Geometry check sheet. Reference: the model listing, model coordinates, mm. Round coordinates to 2 decimals unless told otherwise and drop trailing zeros. Write each loop counter-clockwise with the first axis right and the second up, starting at its lowest first coordinate (ties: lowest second). Pieces come first, ordered by that corner, then holes. Notation, with made-up numbers: M 40,-7 L 68,-7 A18 cw 68,18 Z; hole C 77,11.25 d4. An arc over 180 degrees is marked long. Put each result on its own line as item: value. Start each with the question number.
(1) Section check A-A on x = -110. Record the cut outline in (y, z).
(2) Gauge pin test, flat ends, axial feed: pin 1 (2.5 mm diameter, centred on x = 186, y = -15, fed in from -Z); pin 2 (0.8 mm diameter, centred on y = -16.5, z = 3, fed in from +X); pin 3 (1.2 mm diameter, centred on y = -9.5, z = -4.5, fed in from -X). Record the tip position at first contact, or that the pin passes through.
(3) Material ranges on probe 1 along X at (y, z) = (-21, 2); probe 2 along Y at (x, z) = (120, -0.75), recorded low to high.
from build123d import *

# Parameters (mm, degrees)
F1_DEPTH      = 35
F2_W          = 3
F2_H          = 3
F3_DEPTH      = 187.5
F3_DEPTH_BACK = 187.5


with BuildPart() as f1:
    # F0 (on Front) → F1 (new body)
    with BuildSketch(Plane.XZ):
        Polygon((-226.934456, 2.5), (-226.934456, 0), (-226.934456, -2.5), (-221.934456, -2.5), (-221.934456, -5), (153.065544, -5), (153.065544, -2.5), (158.065544, -2.5), (158.065544, 2.5), (153.065544, 2.5), (153.065544, 5), (-221.934456, 5), (-221.934456, 2.5), align=None)
    extrude(amount=F1_DEPTH)


with BuildPart() as f3:
    # F2 (on Right) → F3 (new body, two sides)
    with BuildSketch(Plane.YZ) as f3_sk:
        with Locations((-32.222062, -1.036781)):
            Rectangle(F2_W, F2_H)
    extrude(amount=F3_DEPTH)
    extrude(f3_sk.sketch, amount=-F3_DEPTH_BACK)


with BuildPart() as f1_1:
    # F4: moved
    add(f1.part.moved(Location((29.4, 1.4, -1))))

    # F5: cut F3
    add(f3.part, mode=Mode.SUBTRACT)


solid = f1_1.part
Answers follow:
1. outline: M -33.6,-6 L 1.4,-6 L 1.4,4 L -33.6,4 L -33.6,0.46 L -30.72,0.46 L -30.72,-2.54 L -33.6,-2.54 Z
2. pin 1: stops at z = -3.5
2. pin 2: stops at x = 182.47
2. pin 3: stops at x = -192.53
3. probe 1: x = -192.53 to 182.47
3. probe 2: y = -30.72 to 1.4
